```python
from build123d import *

# Parameters (mm, degrees)
F0_W     = 330.2
F0_H     = 444.5
F0_W_2   = 317.5
F0_H_2   = 431.8
F1_DEPTH = 38.1
F2_R     = 25.4
F3_D     = 12.7
F3_DEPTH = 165.101
F4_D     = 12.7


with BuildPart() as f1:
    # F0 (on Front) → F1 (new body)
    with BuildSketch(Plane.XZ):
        Rectangle(F0_W, F0_H)
        Rectangle(F0_W_2, F0_H_2, mode=Mode.SUBTRACT)
    extrude(amount=F1_DEPTH)

    # F2
    f2_edges = [f1.edges().sort_by_distance(p)[0] for p in [
        (158.75, -19.05, -215.9),
        (158.75, -19.05, 215.9),
        (-158.75, -19.05, 215.9),
        (-158.75, -19.05, -215.9),
        (165.1, -19.05, 222.25),
        (165.1, -19.05, -222.25),
        (-165.1, -19.05, -222.25),
        (-165.1, -19.05, 222.25),
    ]]
    fillet(f2_edges, radius=F2_R)

    # F3 (through all, one way)
    with BuildSketch(Plane.YZ):
        with Locations((-19.05, 0)):
            Circle(F3_D / 2)
    extrude(amount=-F3_DEPTH, mode=Mode.SUBTRACT)

    # F4 (through all)
    with Locations(Plane(origin=(0, 0, 0), x_dir=(0, 1, 0), z_dir=(-1, 0, 0))):
        with Locations((-19.05, 0)):
            Hole(F4_D / 2)


solid = f1.part
```
For this review, take the finished solid that the model builds, in its own axes (mm). A direction names the side the tool comes from. Coordinates: 2 decimals unless noted, no trailing zeros. Loops run counter-clockwise (first coordinate to the right, second up) from the corner with the lowest first, then second, coordinate; pieces in that order, holes last. Notation, with made-up numbers: (-5.75, 34) - (4.25, 34) arc R21 ccw to (4.25, 59) - close; hole circle Ø10 at (55.25, 17). An arc over 180 degrees is marked (long way). Use one line per item in the form item = value. Start each with the question number.
1) Take a section at B-B (z = -42). State the section outline as (x, y) points.
2) Take a section at A-A (y = -19.05). State the section outline as (x, z) points.
3) Draft analysis for pull direction Z (two halves, no side actions). For faces 3 (the face through (-151.11, -19.32, -208.66)), 4 (the face through (-157.86, -19.32, -214.61)), 5 (the face through (-2, -19, 222.25)), state which applies: released by +Z, released by -Z, zero draft, split by the parting line, or undercut.
4) For faces 1 (the face through (-160, -38.1, 1)), 2 (the face through (151.11, -19.32, -208.66)), list the 3-axis set-ups (+Z, -Z, +X, -X, +Y, -Y) from which the entire face can be reached by the end or side of a thin tool; tool diameter is ignored.
5) To check wall thickness, follow probe 1 along Z at (x, y) = (81, -4); probe 2 along X at (y, z) = (-16.5, -48.5); probe 3 along Z at (x, y) = (137, -31). State the ranges of each line that lie inside material, in increasing order. Write a range as from..to.
6) For pin 1 (10 mm diameter, centred on y = -19.05, z = 0, fed in from -X), flat-tipped, find the tip position at first contact; note if it passes through.
7) Take a section at C-C (x = -21). State the section outline as (y, z) points.
From the geometry:
q1.outline = (-165.1, -38.1) - (-158.75, -38.1) - (-158.75, 0) - (-165.1, 0) - close; (158.75, -38.1) - (165.1, -38.1) - (165.1, 0) - (158.75, 0) - close
q2.outline = (-165.1, -196.85) arc R25.4 ccw to (-139.7, -222.25) - (139.7, -222.25) arc R25.4 ccw to (165.1, -196.85) - (165.1, -6.35) - (158.75, -6.35) - (158.75, -190.5) arc R25.4 cw to (133.35, -215.9) - (-133.35, -215.9) arc R25.4 cw to (-158.75, -190.5) - (-158.75, -6.35) - (-165.1, -6.35) - close; (-165.1, 6.35) - (-158.75, 6.35) - (-158.75, 190.5) arc R25.4 cw to (-133.35, 215.9) - (133.35, 215.9) arc R25.4 cw to (158.75, 190.5) - (158.75, 6.35) - (165.1, 6.35) - (165.1, 196.85) arc R25.4 ccw to (139.7, 222.25) - (-139.7, 222.25) arc R25.4 ccw to (-165.1, 196.85) - close
q3.face_3 = undercut
q3.face_4 = released by -Z
q3.face_5 = released by +Z
q4.face_1 = +Z, -Z, +X, -X, -Y
q4.face_2 = +Y, -Y
q5.probe_1 = -222.25..-215.9, 215.9..222.25
q5.probe_2 = -165.1..-158.75, 158.75..165.1
q5.probe_3 = -222.25..-215.64, 215.64..222.25
q6.pin_1 = through
q7.outline = (-38.1, -222.25) - (0, -222.25) - (0, -215.9) - (-38.1, -215.9) - close; (-38.1, 215.9) - (0, 215.9) - (0, 222.25) - (-38.1, 222.25) - close
